Geometry check sheet. Reference: the model listing, model coordinates, mm. Face numbers are marked on the shaded views. A direction names the side the tool comes from. Round coordinates to 2 decimals unless told otherwise and drop trailing zeros. Order: outer loops, then holes, each group sorted by start corner. A loop starts at its lowest first (then second) coordinate and runs counter-clockwise, first axis right, second up.
(1) Cross-section at A-A on y = 0. Enter the section's corners in (x, z), and give its area (3 significant figures).
(2) Cross-section at B-B on z = -6.5. Enter the section's corners in (x, y).
(3) Cross-section at D-D on x = 47.5. Enter the section's corners in (y, z).
(4) Gauge pin test, flat ends, axial feed: P1, Ø6, axis at x = 17, y = 5, coming from the +Z side; P2, Ø5, axis at x = 5.5, z = 2.5, coming from the -Y side; P3, Ø1.5, axis at x = 24, y = -5, coming from the +Z side; P4, Ø8, axis at x = 43.5, z = 0.5, coming from the -Y side. Record the tip position at first contact, or that the pin passes through.
(5) Cross-section at C-C on z = 4.75. Enter the section's corners in (x, y).
(6) Set-up check for the marked faces 1 and 2: record each of +Z, -Z, +X, -X, +Y, -Y from which the full face is reachable in a straight line by a thin tool's end or side.
(7) Thickness scan on L1, parallel to X at y = 0, z = -5.5; L2, parallel to Z at x = 7.5, y = 0; L3, parallel to Y at x = 12.5, z = -2. Record the ranges inside material, lowest first.
from build123d import *

# Parameters (mm, degrees)
F0_R     = 7.5
F1_DEPTH = 25
F2_R     = 8.25
F3_DEPTH = 25
F4_R     = 1.75
F5_DEPTH = 25


with BuildPart() as f1:
    # F0 (on Right) → F1 (new body)
    with BuildSketch(Plane.YZ):
        Circle(F0_R)
    extrude(amount=F1_DEPTH)

    # F2 (on face) → F3 (join)
    with BuildSketch(Plane.YZ.offset(25)):
        Circle(F2_R)
    extrude(amount=F3_DEPTH)

    # F4 (on Top) → F5 (cut)
    with BuildSketch(Plane.XY):
        with Locations((12.5, 0)):
            Circle(F4_R)
    extrude(amount=-F5_DEPTH, mode=Mode.SUBTRACT)


solid = f1.part
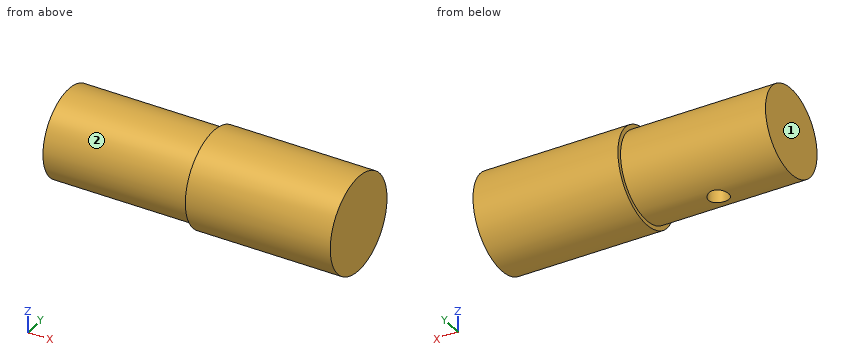
Found:
1. outline: (0, -7.5) - (10.75, -7.5) - (10.75, 0) - (14.25, 0) - (14.25, -7.5) - (25, -7.5) - (25, -8.25) - (50, -8.25) - (50, 8.25) - (25, 8.25) - (25, 7.5) - (0, 7.5) - close
1. area: 761 mm2
2. outline: (0, -3.74) - (25, -3.74) - (25, -5.08) - (50, -5.08) - (50, 5.08) - (25, 5.08) - (25, 3.74) - (0, 3.74) - close; hole circle Ø3.5 at (12.5, 0)
3. outline: circle Ø16.5 at (0, 0)
4. P1: stops at z = 7.23
4. P2: stops at y = -7.5
4. P3: stops at z = 6.18
4. P4: stops at y = -8.25
5. outline: (0, -5.8) - (25, -5.8) - (25, -6.75) - (50, -6.75) - (50, 6.75) - (25, 6.75) - (25, 5.8) - (0, 5.8) - close
6. face 1: +Z, -Z, -X, +Y, -Y
6. face 2: -X
7. L1: x = 0 to 10.75, 14.25 to 50
7. L2: z = -7.5 to 7.5
7. L3: y = -7.23 to -1.75, 1.75 to 7.23
